Build history of the part. All positions in model axes, mm. Face numbers are marked on the shaded views. A direction names the side the tool comes from. Round coordinates to 2 decimals unless told otherwise and drop trailing zeros. Write each loop counter-clockwise with the first axis right and the second up, starting at its lowest first coordinate (ties: lowest second). Pieces come first, ordered by that corner, then holes. Notation, with made-up numbers: M 27,8.25 L 50,8.25 A9 cw 50,25.25 Z; hole C 20,-21 d11. An arc over 180 degrees is marked long. Write item = value, one per line.
from build123d import *

# Parameters (mm, degrees)
F0_W     = 0.975
F0_H     = 3.05
F0_H_2   = 10
F0_R     = 1.8
F1_DEPTH = 5
F2_DEPTH = 1.5
F3_DEPTH = 7.1


with BuildPart() as f1:
    # F0 (on Top) → F1 (new body)
    with BuildSketch(Plane.XY):
        Polygon((5, -9.1), (5, -8.05), (4.025, -8.05), (-4.025, -8.05), (-5, -8.05), (-5, -9.1), align=None)
        with Locations((4.5125, -6.525)):
            Rectangle(F0_W, F0_H)
        Polygon((4.025, 5), (4.025, 8.05), (-4.025, 8.05), (-4.025, 5), (-4.025, -5), (-4.025, -8.05), (4.025, -8.05), (4.025, -5), align=None)
        with BuildLine():
            ThreePointArc((-2.8, 3), (0, 5.8), (2.8, 3))
            Line((2.8, 3), (2.8, 0))
            Line((2.8, 0), (2.8, -3))
            ThreePointArc((2.8, -3), (0, -5.8), (-2.8, -3))
            Line((-2.8, -3), (-2.8, 0))
            Line((-2.8, 0), (-2.8, 3))
        make_face(mode=Mode.SUBTRACT)
        with Locations((-4.5125, -6.525)):
            Rectangle(F0_W, F0_H)
        with Locations((-4.5125, 0)):
            Rectangle(F0_W, F0_H_2)
        with Locations((4.5125, 0)):
            Rectangle(F0_W, F0_H_2)
        with Locations((4.5125, 6.525)):
            Rectangle(F0_W, F0_H)
        Polygon((5, 8.05), (5, 9.1), (-5, 9.1), (-5, 8.05), (-4.025, 8.05), (4.025, 8.05), align=None)
        with BuildLine():
            Line((2.8, 0), (2.8, 3))
            ThreePointArc((2.8, 3), (0, 5.8), (-2.8, 3))
            Line((-2.8, 3), (-2.8, 0))
            Line((-2.8, 0), (-2.8, -3))
            ThreePointArc((-2.8, -3), (0, -5.8), (2.8, -3))
            Line((2.8, -3), (2.8, 0))
        make_face()
        with Locations((0, -3)):
            Circle(F0_R, mode=Mode.SUBTRACT)
        with Locations((0, 3)):
            Circle(F0_R, mode=Mode.SUBTRACT)
        with Locations((-4.5125, 6.525)):
            Rectangle(F0_W, F0_H)
    extrude(amount=F1_DEPTH)

    # F0 (on Top) → F2 (cut)
    with BuildSketch(Plane.XY):
        with BuildLine():
            Line((2.8, 0), (2.8, 3))
            ThreePointArc((2.8, 3), (0, 5.8), (-2.8, 3))
            Line((-2.8, 3), (-2.8, 0))
            Line((-2.8, 0), (-2.8, -3))
            ThreePointArc((-2.8, -3), (0, -5.8), (2.8, -3))
            Line((2.8, -3), (2.8, 0))
        make_face()
        with Locations((0, -3)):
            Circle(F0_R, mode=Mode.SUBTRACT)
        with Locations((0, 3)):
            Circle(F0_R, mode=Mode.SUBTRACT)
    extrude(amount=F2_DEPTH, mode=Mode.SUBTRACT)

    # F0 (on Top) → F3 (join)
    with BuildSketch(Plane.XY):
        with Locations((-4.5125, 0)):
            Rectangle(F0_W, F0_H_2)
        Polygon((5, -9.1), (5, -8.05), (4.025, -8.05), (-4.025, -8.05), (-5, -8.05), (-5, -9.1), align=None)
        with Locations((4.5125, 0)):
            Rectangle(F0_W, F0_H_2)
        Polygon((5, 8.05), (5, 9.1), (-5, 9.1), (-5, 8.05), (-4.025, 8.05), (4.025, 8.05), align=None)
    extrude(amount=F3_DEPTH)


solid = f1.part
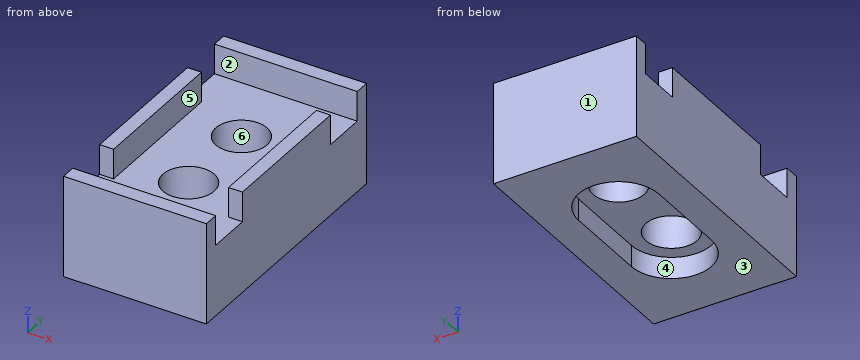
1. Tool access for the marked faces 4, 5 and 6: list every direction of +Z, -Z, +X, -X, +Y, -Y with a clear straight run to the whole face (end or side of a thin tool).
Responses:
face_4 = -Z
face_5 = +Z
face_6 = +Z, -Z
2. Band-saw the part on B-B (z = 1). List the corners of the cut face in (x, y).
Responses:
outline = M -5,-9.1 L 5,-9.1 L 5,9.1 L -5,9.1 Z; hole M -2.8,-3 A2.8 ccw 2.8,-3 L 2.8,3 A2.8 ccw -2.8,3 Z
3. Probe probe 1 along Y at (x, z) = (0, 2.35); probe 2 along X at (y, z) = (1, 6.75) (3 decimals); probe 3 along Z at (x, y) = (2.75, -0.5). List the from-to ranges inside material, lowest first.
Responses:
probe_1 = -9.1 to -4.8, -1.2 to 1.2, 4.8 to 9.1
probe_2 = -5 to -4.025, 4.025 to 5
probe_3 = 1.5 to 5
4. Mould opens along Y. For the marked faces 1, 2 and 3 say: pulls with the +Y half, pulls with the -Y half, needs draft (parallel to the pull), parting line crosses it, or undercut.
Responses:
face_1 = pulls with the +Y half
face_2 = undercut
face_3 = needs draft
5. Flat gauge pin, fed straight in: pin 1 (4 mm diameter, centred on x = 0, y = 4, fed in from +Z). Where does the tip first touch, or does it go through?
Responses:
pin_1 = 5
6. Band-saw the part on A-A (x = 0). List the corners of the cut face in (y, z), plus the area to 3 significant figures.
Responses:
outline = M -9.1,0 L -5.8,0 L -5.8,1.5 L -4.8,1.5 L -4.8,5 L -8.05,5 L -8.05,7.1 L -9.1,7.1 Z; M -1.2,1.5 L 1.2,1.5 L 1.2,5 L -1.2,5 Z; M 4.8,1.5 L 5.8,1.5 L 5.8,0 L 9.1,0 L 9.1,7.1 L 8.05,7.1 L 8.05,5 L 4.8,5 Z
area = 52.8 mm²
7. Band-saw the part on C-C (y = -2.75). List the corners of the cut face in (x, z) (3 decimals).
Responses:
outline = M -5,0 L -2.8,0 L -2.8,1.5 L -1.783,1.5 L -1.783,5 L -4.025,5 L -4.025,7.1 L -5,7.1 Z; M 1.783,1.5 L 2.8,1.5 L 2.8,0 L 5,0 L 5,7.1 L 4.025,7.1 L 4.025,5 L 1.783,5 Z
8. Band-saw the part on D-D (z = 5.75). List the corners of the cut face in (x, y) (3 decimals), plus the area to 3 significant figures.
Responses:
outline = M -5,-9.1 L 5,-9.1 L 5,-8.05 L -5,-8.05 Z; M -5,-5 L -4.025,-5 L -4.025,5 L -5,5 Z; M -5,8.05 L 5,8.05 L 5,9.1 L -5,9.1 Z; M 4.025,-5 L 5,-5 L 5,5 L 4.025,5 Z
area = 40.5 mm²
